Here's how the part is built. I have some questions about the finished solid (model axes, mm). Face numbers are marked on the shaded views. A direction names the side the tool comes from. Round coordinates to 2 decimals unless told otherwise and drop trailing zeros. Loops run counter-clockwise (first coordinate to the right, second up) from the corner with the lowest first, then second, coordinate; pieces in that order, holes last. Notation, with made-up numbers: M -5.75,57.25 L 34.25,57.25 A6 cw 34.25,65.25 Z; hole C -28,82 d10. An arc over 180 degrees is marked long. Answer as CSV lines item,"result".
Autodesk Inventor part; units mm, degrees
ref_plane "YZ Plane" through (0, 0, 0) normal (1, 0, 0) x (0, 1, 0)
ref_plane "XZ Plane" through (0, 0, 0) normal (0, 1, 0) x (-1, 0, 0)
ref_plane "XY Plane" through (0, 0, 0) normal (0, 0, 1) x (1, 0, 0)
sketch "Sketch1" plane through (0, 0, 0) normal (0, 0, 1) x (1, 0, 0)
  line L0 (-4.5, 15) -> (4.5, 15)
  line L1 (4.5, 15) -> (4.5, -15)
  line L2 (4.5, -15) -> (-4.5, -15)
  line L3 (-4.5, -15) -> (-4.5, 15)
  line L4 (-4.5, 15) -> (4.5, -15) construction
  line L5 (4.5, 15) -> (-4.5, -15) construction
  circle A0 centre (0, 15) radius 4.5
  circle A1 centre (0, -15) radius 4.5
  point P0 (0, 0)
  point P1 (-4.5, 15)
  point P2 (-4.5, -15)
  dimension "d0" = 9
  dimension "d1" = 30
extrude "Extrusion1" add sketch "Sketch1" against normal blind 5
sketch "Sketch3" plane through (0, 0, -5) normal (0, 0, -1) x (-1, 0, 0)
  line L0 (4.5, -15) -> (4.5, 15)
  arc A0 (4.5, 15) -> (-4.5, 15) centre (0, 15) ccw
  line L1 (-4.5, 15) -> (-4.5, -15)
  arc A1 (-4.5, -15) -> (4.5, -15) centre (0, -15) ccw
  line L2 (-9.5, -15) -> (-9.5, 15)
  arc A2 (9.5, 15) -> (-9.5, 15) centre (0, 15) ccw
  line L3 (9.5, 15) -> (9.5, -15)
  arc A3 (-9.5, -15) -> (9.5, -15) centre (0, -15) ccw
  point P0 (0, 0)
  dimension "d9" = 5
extrude "Extrusion3" add sketch "Sketch3" against normal blind 2
sketch "Sketch5" plane through (0, 0, -5) normal (0, 0, -1) x (-1, 0, 0)
  line L0 (-9.5, 15) -> (-9.5, -15)
  arc A0 (-9.5, -15) -> (9.5, -15) centre (0, -15) ccw
  line L1 (9.5, -15) -> (9.5, 15)
  arc A1 (9.5, 15) -> (-9.5, 15) centre (0, 15) ccw
  circle A2 centre (0, 12.9469) radius 2.5
  circle A3 centre (0, -13.0531) radius 2.5
  point P0 (0, 0)
  dimension "d12" = 26
  dimension "d13" = 5
extrude "Extrusion4" cut sketch "Sketch5" against normal blind 1.8 contours A2 | A3
chamfer "Chamfer1" distance 0.5 angle 45 2 edges at (2.5, 12.9469, -5) (2.5, -13.0531, -5)
fillet "Fillet2" radius 0.5 4 edges at (0, 19.5, 0) (-4.5, 0, 0) (0, -19.5, 0) (4.5, 0, 0)
properties part number "KLEP_KNOPPEN"
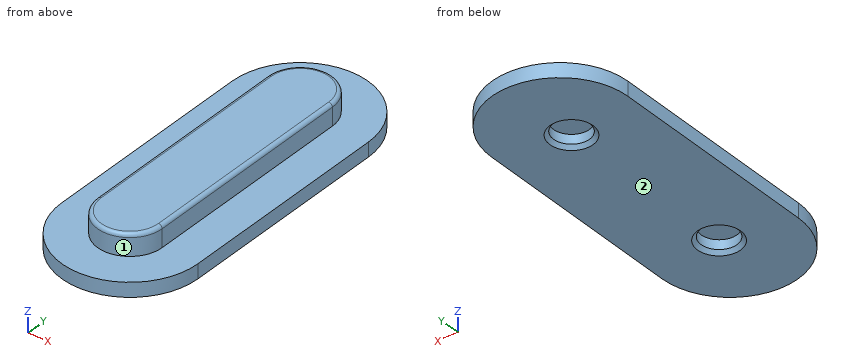
1. If I drill on line 1 (Y direction, x = 0, z = -3.7); line 2 (Y direction, x = -1, z = -3.4); line 3 (X direction, y = 8, z = -1.35), over which ranges is the centre line in solid material (lowest first)? Write a range as [from, to].
Evaluation:
line 1,"y = [-24.5, -15.55], [-10.55, 10.45], [15.45, 24.5]"
line 2,"y = [-24.45, -15.34], [-10.76, 10.66], [15.24, 24.45]"
line 3,"x = [-4.5, 4.5]"
2. Which directions (+Z, -Z, +X, -X, +Y, -Y) give clear straight access to the entire face, cutting with the end or side of a thin tool? Please do the marked faces 1 and 2.
Evaluation:
face 1,"+Z, -Y"
face 2,"-Z, +X, -X, +Y, -Y"
3. I want a section at D-D, the plane z = -3.7. Please give me the cut outline in (x, y), and give its area (3 significant figures).
Evaluation:
outline,"M -9.5,-15 A9.5 ccw 9.5,-15 L 9.5,15 A9.5 ccw -9.5,15 Z; hole C 0,-13.05 d5; hole C 0,12.95 d5"
area,"814 mm²"
4. I want a section at A-A, the plane y = 4. Please give me the cut outline in (x, z), and give its area (3 significant figures).
Evaluation:
outline,"M -9.5,-5 L 9.5,-5 L 9.5,-3 L 4.5,-3 L 4.5,-0.5 A0.5 ccw 4,0 L -4,0 A0.5 ccw -4.5,-0.5 L -4.5,-3 L -9.5,-3 Z"
area,"64.9 mm²"
5. I want a section at C-C, the plane z = -1.05. Please give me the cut outline in (x, y), and give its area (3 significant figures).
Evaluation:
outline,"M -4.5,-15 A4.5 ccw 4.5,-15 L 4.5,15 A4.5 ccw -4.5,15 Z"
area,"334 mm²"
6. For P1, Ø2, axis at x = 4, y = -18.5, coming from the +Z side; P2, Ø4, axis at x = 6, y = -16.5, coming from the +Z side; P3, Ø1, axis at x = 1, z = -4, coming from the +Y side; P4, Ø3, axis at y = -4.5, z = -2.5, coming from the -X side, each with a flat end and sliding along its axis, tell me the tip position at first contact or that it passes through.
Evaluation:
P1,"stops at z = -0.11"
P2,"stops at z = -0.04"
P3,"stops at y = 24.49"
P4,"stops at x = -9.5"
7. I want a section at B-B, the plane x = 0. Please give me the cut outline in (y, z), and give its area (3 significant figures).
Evaluation:
outline,"M -24.5,-5 L -16.05,-5 L -15.55,-4.5 L -15.55,-3.2 L -10.55,-3.2 L -10.55,-4.5 L -10.05,-5 L 9.95,-5 L 10.45,-4.5 L 10.45,-3.2 L 15.45,-3.2 L 15.45,-4.5 L 15.95,-5 L 24.5,-5 L 24.5,-3 L 19.5,-3 L 19.5,-0.5 A0.5 ccw 19,0 L -19,0 A0.5 ccw -19.5,-0.5 L -19.5,-3 L -24.5,-3 Z"
area,"196 mm²"
